Source: CAD feature listing. Evaluate the final solid. Frame: model axes, mm. A direction names the side the tool comes from. Give positions to 0.01 mm unless a question says otherwise; leave off trailing zeros. Loops run counter-clockwise (first coordinate to the right, second up) from the corner with the lowest first, then second, coordinate; pieces in that order, holes last. Notation, with made-up numbers: M 4.5,27 L 21.5,27 A18 ccw 21.5,59 Z; hole C -33.5,48 d6. An arc over 180 degrees is marked long. Answer in a Markdown table with one row per item.
```python
from build123d import *

# Parameters (mm, degrees)
SKETCH2_R           = 18.85
SKETCH2_R_2         = 1.350069841
BOSS_EXTRUDE1_DEPTH = 8
SKETCH3_R           = 30
SKETCH3_R_2         = 17.600030795
BOSS_EXTRUDE2_DEPTH = 8
SKETCH4_R           = 2.9
BOSS_EXTRUDE3_DEPTH = 2
SKETCH6_R           = 5
BOSS_EXTRUDE4_DEPTH = 3
SKETCH5_R           = 3
CUT_EXTRUDE1_DEPTH  = 3
SKETCH7_R           = 25
CUT_EXTRUDE2_DEPTH  = 8
FILLET1_R           = 5


with BuildPart() as part:
    # Sketch2 → Boss-Extrude1 (new body)
    with BuildSketch(Plane.XY.offset(10)):
        Circle(SKETCH2_R)
        with Locations((7.824268806, 11.301452471)):
            Circle(SKETCH2_R_2, mode=Mode.SUBTRACT)
        with Locations((3.924268806, 11.301452471)):
            Circle(SKETCH2_R_2, mode=Mode.SUBTRACT)
        with Locations((0.024268806, 11.301452471)):
            Circle(SKETCH2_R_2, mode=Mode.SUBTRACT)
        with Locations((-3.875731194, 11.301452471)):
            Circle(SKETCH2_R_2, mode=Mode.SUBTRACT)
        with Locations((-7.775731194, 11.301452471)):
            Circle(SKETCH2_R_2, mode=Mode.SUBTRACT)
        with Locations((9.749100056, 5.629684708)):
            Circle(SKETCH2_R_2, mode=Mode.SUBTRACT)
    extrude(amount=BOSS_EXTRUDE1_DEPTH)

    # Sketch3 → Boss-Extrude2 (add)
    with BuildSketch(Plane.XY.offset(18)):
        Circle(SKETCH3_R)
        Circle(SKETCH3_R_2, mode=Mode.SUBTRACT)
    extrude(amount=-BOSS_EXTRUDE2_DEPTH)

    # Sketch4 → Boss-Extrude3 (add)
    with BuildSketch(Plane.XY.offset(18)):
        with Locations((0, 25)):
            Circle(SKETCH4_R)
        with Locations((21.650635095, -12.5)):
            Circle(SKETCH4_R)
        with Locations((-21.650635095, -12.5)):
            Circle(SKETCH4_R)
    extrude(amount=BOSS_EXTRUDE3_DEPTH)

    # Sketch6 → Boss-Extrude4 (add)
    with BuildSketch(Plane(origin=(0, 0, 10), x_dir=(-1, 0, 0), z_dir=(0, 0, -1))):
        with Locations((0, 30)):
            Circle(SKETCH6_R)
        with Locations((25.980762114, -15)):
            Circle(SKETCH6_R)
        with Locations((-25.980762114, -15)):
            Circle(SKETCH6_R)
    extrude(amount=-BOSS_EXTRUDE4_DEPTH)

    # Sketch5 → Cut-Extrude1 (cut)
    with BuildSketch(Plane(origin=(0, 0, 10), x_dir=(-1, 0, 0), z_dir=(0, 0, -1))):
        with Locations((0, 25)):
            Circle(SKETCH5_R)
        with Locations((21.650635095, -12.5)):
            Circle(SKETCH5_R)
        with Locations((-21.650635095, -12.5)):
            Circle(SKETCH5_R)
    extrude(amount=-CUT_EXTRUDE1_DEPTH, mode=Mode.SUBTRACT)

    # Sketch7 → Cut-Extrude2 (cut)
    with BuildSketch(Plane(origin=(0, 0, 10), x_dir=(-1, 0, 0), z_dir=(0, 0, -1))):
        with Locations((-35.980083702, 21.666415873)):
            Circle(SKETCH7_R)
        with Locations((36.753708406, 20.32645858)):
            Circle(SKETCH7_R)
        with Locations((-0.773624703, -41.992874453)):
            Circle(SKETCH7_R)
    extrude(amount=-CUT_EXTRUDE2_DEPTH, mode=Mode.SUBTRACT)

    # Fillet1
    fillet1_edges = [part.edges().sort_by_distance(p)[0] for p in [
        (29.888839754, -2.580166302, 14),
        (11.700383981, 27.624283062, 14),
        (-12.709930313, 27.174577668, 14),
        (-29.773522884, -3.679311769, 14),
        (-17.178909441, -24.594411366, 14),
        (18.073138902, -23.944971293, 14),
    ]]
    fillet(fillet1_edges, radius=FILLET1_R)


solid = part.part
```
Q1. Contact query for flat-ended pins moving along their axis: pin 1 Ø1.8 at (x, y) = (-20.5, -13.5) entering from -Z; pin 2 Ø1.5 at (y, z) = (-8, 14.5) entering from +X; pin 3 Ø6 at (y, z) = (-10.5, 15.5) entering from +X. Output: stop coordinate, or through.
Values follow:
| item | result |
|---|---|
| pin 1 | z = 13 |
| pin 2 | x = 29.11 |
| pin 3 | x = 30.09 |
Q2. Reachability of faces 1 (the cylindrical face through (18.88, -13.65, 11.48)), 2 (the cylindrical face through (-18.97, -13.61, 18.99)), 3 (the cylindrical face through (-0.268, 9.983, 13.944)) from +Z, -Z, +X, -X, +Y, -Y: full face, straight path, thin tool, end or side. Return the list, or none.
Values follow:
| item | result |
|---|---|
| face 1 | -Z |
| face 2 | +Z |
| face 3 | +Z, -Z |
Q3. Mould query, pull axis X, two halves, no side actions, for faces 4 (the cylindrical face through (0, 30, 15)), 5 (the cylindrical face through (0.65, 22.07, 11.48)), 6 (the flat face through (-22, -12, 20)). Classes: +X half, -X half, draft (parallel to the pull), parting line (faces both ways), or undercut.
Values follow:
| item | result |
|---|---|
| face 4 | parting line |
| face 5 | undercut |
| face 6 | draft |
Q4. Section query D-D (z = 11.5). Give the number of separate pieces and of enclosed holes in the cut face, plus the area to 3 significant figures.
Values follow:
| item | result |
|---|---|
| separate pieces | 1 |
| enclosed holes | 9 |
| area | 1,870 mm^2 |
Q5. Section query C-C (y = -14.5). Output: boundary loops of the cut face in (x, z), plus the area to 3 significant figures.
Values follow:
| item | result |
|---|---|
| outline | M -30.96,10 L -23.89,10 L -23.89,13 L -19.41,13 L -19.41,10 L 19.41,10 L 19.41,13 L 23.89,13 L 23.89,10 L 30.96,10 L 30.96,13 L 26.26,13 L 26.26,18 L 23.75,18 L 23.75,20 L 19.55,20 L 19.55,18 L -19.55,18 L -19.55,20 L -23.75,20 L -23.75,18 L -26.26,18 L -26.26,13 L -30.96,13 Z |
| area | 438 mm^2 |
Q6. Section query A-A (x = 0). Output: boundary loops of the cut face in (y, z).
Values follow:
| item | result |
|---|---|
| outline | M -17,10 L 9.95,10 L 9.95,18 L -17,18 Z; M 12.65,10 L 22,10 L 22,13 L 28,13 L 28,10 L 35,10 L 35,13 L 30,13 L 30,18 L 27.9,18 L 27.9,20 L 22.1,20 L 22.1,18 L 12.65,18 Z |
Q7. Ray query, probe 1 along Z at (x, y) = (-11.5, 23); probe 2 along Y at (x, z) = (9, 15); probe 3 along X at (y, z) = (5, 16.25). Return the intervals inside material, ascending. Write a range as from..to.
Values follow:
| item | result |
|---|---|
| probe 1 | 10..18 |
| probe 2 | -18.39..4.51, 6.75..10.64, 11.97..28.31 |
| probe 3 | -17..8.55, 10.94..17.35 |
Q8. Section query B-B (z = 18.75). Output: boundary loops of the cut face in (x, y), plus the area to 3 significant figures.
Values follow:
| item | result |
|---|---|
| outline | C -21.65,-12.5 d5.8; C 0,25 d5.8; C 21.65,-12.5 d5.8 |
| area | 79.3 mm^2 |
